Build history of the part. All positions in model axes, mm. Round coordinates to 2 decimals unless told otherwise and drop trailing zeros. Return JSON: item names as keys, results as strings.
from build123d import *

# Parameters (mm, degrees)
F_44_0_086_DIAMETER_HOLE1_D = 2.1844
SCREW_PASSTHROUGHS_COUNT    = 12


with BuildPart() as part:
    # Sketch1 → Main (revolve)
    with BuildSketch(Plane.XY):
        with BuildLine():
            Line((-76.5175, 0), (-82.042, 0))
            ThreePointArc((-82.042, 0), (-82.266506403, 0.092993597), (-82.3595, 0.3175))
            Line((-82.3595, 0.3175), (-82.3595, 2.8575))
            ThreePointArc((-82.3595, 2.8575), (-82.266506403, 3.082006403), (-82.042, 3.175))
            Line((-82.042, 3.175), (-76.5175, 3.175))
            ThreePointArc((-76.5175, 3.175), (-76.292993597, 3.082006403), (-76.2, 2.8575))
            Line((-76.2, 2.8575), (-76.2, 0.3175))
            ThreePointArc((-76.2, 0.3175), (-76.292993597, 0.092993597), (-76.5175, 0))
        make_face()
    revolve(axis=Axis((0, 55, 0), (0, -1, 0)))

    # #44 (0.086) Diameter Hole1 (through all)
    with Locations(Plane(origin=(0, 0, 0), x_dir=(-1, 0, 0), z_dir=(0, -1, 0))):
        with Locations((79.27975, 0)):
            f_44_0_086_diameter_hole1 = Hole(F_44_0_086_DIAMETER_HOLE1_D / 2)

    # Screw Passthroughs: #44 (0.086) Diameter Hole1 ×12 about axis
    screw_passthroughs_axis = Axis((0, 0, 0), (0, 1, 0))
    for i in range(1, SCREW_PASSTHROUGHS_COUNT):
        add(f_44_0_086_diameter_hole1.rotate(screw_passthroughs_axis, i * 360 / SCREW_PASSTHROUGHS_COUNT), mode=Mode.SUBTRACT)


solid = part.part
Q1. Two-plate mould, pull along Z, no slides. Class faces 1 (the cylindrical face through (-76.08, 1.61, 31.54)), 2 (the cylindrical face through (60.47, 1.57, 46.367)), 3 (the flat face through (-25, 0, 73)): +Z half, -Z half, draft (parallel to the pull), parting line (faces both ways), or undercut.
Verdict:
{"face 1": "parting line", "face 2": "undercut", "face 3": "draft"}
Q2. Wall check: L1, parallel to X at y = 1.9, z = -40.5; L2, parallel to Z at x = 68, y = 2.85; L3, parallel to Z at x = 45.5, y = 0.6. Give the ranges that are in metal, low to high.
Verdict:
{"L1": "x = -71.71 to -69.33, -67.99 to -64.55, 64.55 to 67.99, 69.33 to 71.71", "L2": "z = -46.47 to -40.51, -38.77 to -34.39, 34.39 to 38.77, 40.51 to 46.47", "L3": "z = -68.65 to -61.12, 61.12 to 68.65"}
Q3. Pin check, flat tips, straight feed: pin 1 Ø1.7 at (x, z) = (-39.64, 68.66) entering from -Y; pin 2 Ø1 at (y, z) = (2.5, 1.5) entering from -X; pin 3 Ø2.5 at (x, z) = (39.64, 68.66) entering from +Y (3 decimals). Stop position of each tip, or through.
Verdict:
{"pin 1": "passes through", "pin 2": "stops at x = -82.35", "pin 3": "stops at y = 3.175"}
Q4. Saw through at A-A on y = 2. Count the separate pieces of the cut face and the enclosed holes in it, then the cut area to 3 significant figures.
Verdict:
{"separate pieces": "1", "enclosed holes": "13", "area": "3,020 mm²"}
